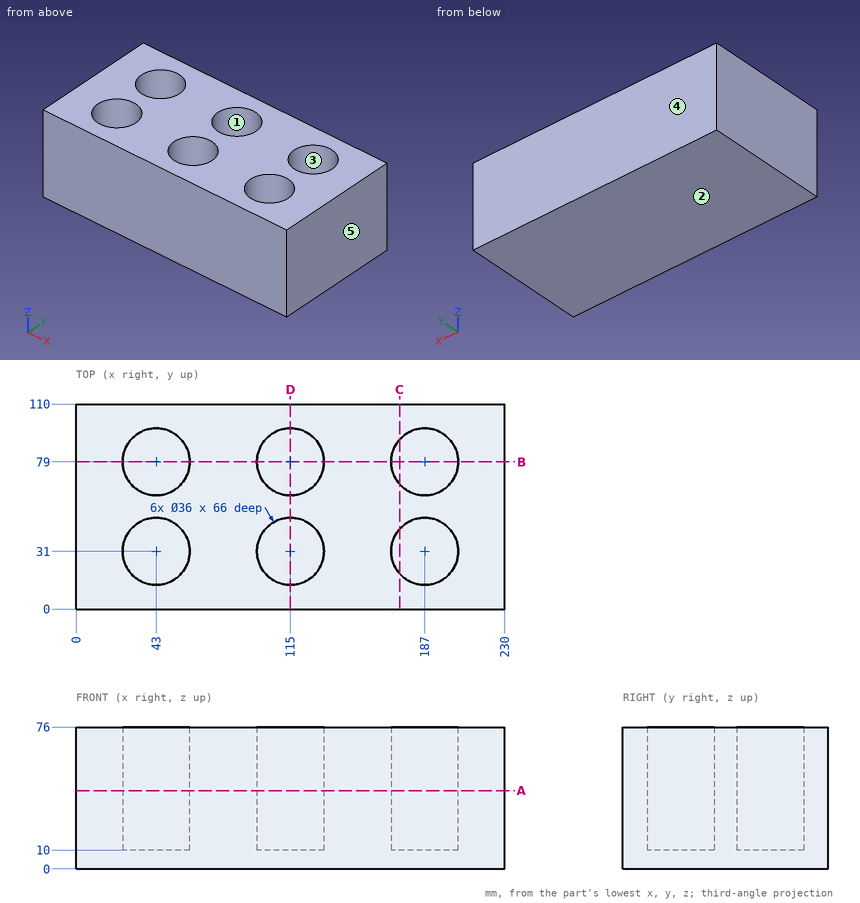
Input: dimensioned drawing with shaded views. Units: mm. Origin: part minimum x, y, z. A direction names the side the tool comes from. Round coordinates to 2 decimals unless told otherwise and drop trailing zeros. Loops run counter-clockwise (first coordinate to the right, second up) from the corner with the lowest first, then second, coordinate; pieces in that order, holes last. Notation, with made-up numbers: M 50,4 L 81,4 A19 cw 81,20 Z; hole C -29,-23.5 d9. An arc over 180 degrees is marked long. Answer in a Markdown table with one row per item. Add a question column.
1. Section A-A (z = 42). Output: boundary loops of the cut face in (x, y).
2. Section B-B (y = 79). Output: boundary loops of the cut face in (x, z).
3. Mould query, pull axis Y, two halves, no side actions, for the marked faces 3, 4 and 5. Classes: released by +Y, released by -Y, zero draft, split by the parting line, or undercut.
4. Set-up query: the marked faces 1 and 2. Return all of +Z, -Z, +X, -X, +Y, -Y with unobstructed straight access to the full face (end or side cutting, diameter ignored); none if empty.
5. Contact query for flat-ended pins moving along their axis: pin 1 (6 mm diameter, centred on x = 122, z = 12.5, fed in from -Y); pin 2 (18 mm diameter, centred on x = 184.5, y = 82, fed in from +Z). Output: stop coordinate, or through.
6. Ray query, probe 1 along Y at (x, z) = (187, 60.5); probe 2 along X at (y, z) = (31, 31); probe 3 along X at (y, z) = (84, 50). Return the intervals inside material, ascending.
7. Section C-C (x = 173.5). Output: boundary loops of the cut face in (y, z), and give its area (3 significant figures).
8. Section D-D (x = 115). Output: boundary loops of the cut face in (y, z), and give its area (3 significant figures).
Values follow:
| question | item | result |
|---|---|---|
| 1 | outline | M 0,0 L 230,0 L 230,110 L 0,110 Z; hole C 43,31 d36; hole C 43,79 d36; hole C 115,31 d36; hole C 115,79 d36; hole C 187,31 d36; hole C 187,79 d36 |
| 2 | outline | M 0,0 L 230,0 L 230,76 L 205,76 L 205,10 L 169,10 L 169,76 L 133,76 L 133,10 L 97,10 L 97,76 L 61,76 L 61,10 L 25,10 L 25,76 L 0,76 Z |
| 3 | face 3 | undercut |
| 3 | face 4 | released by +Y |
| 3 | face 5 | zero draft |
| 4 | face 1 | +Z |
| 4 | face 2 | -Z, +X, -X, +Y, -Y |
| 5 | pin 1 | y = 0 |
| 5 | pin 2 | z = 10 |
| 6 | probe 1 | 0 to 13, 49 to 61, 97 to 110 |
| 6 | probe 2 | 0 to 25, 61 to 97, 133 to 169, 205 to 230 |
| 6 | probe 3 | 0 to 25.71, 60.29 to 97.71, 132.29 to 169.71, 204.29 to 230 |
| 7 | outline | M 0,0 L 110,0 L 110,76 L 90.91,76 L 90.91,10 L 67.09,10 L 67.09,76 L 42.91,76 L 42.91,10 L 19.09,10 L 19.09,76 L 0,76 Z |
| 7 | area | 5,220 mm^2 |
| 8 | outline | M 0,0 L 110,0 L 110,76 L 97,76 L 97,10 L 61,10 L 61,76 L 49,76 L 49,10 L 13,10 L 13,76 L 0,76 Z |
| 8 | area | 3,610 mm^2 |
